CAD build for the part. Positions are in the model's coordinates, mm. Face numbers are marked on the shaded views. A direction names the side the tool comes from. Round coordinates to 2 decimals unless told otherwise and drop trailing zeros. Order: outer loops, then holes, each group sorted by start corner. A loop starts at its lowest first (then second) coordinate and runs counter-clockwise, first axis right, second up. Notation, with made-up numbers: M 8,26.5 L 22,26.5 A20 ccw 22,49.5 Z; hole C -35,39.5 d2. An arc over 180 degrees is marked long. Put each result on its own line as item: value.
```python
from build123d import *

# Parameters (mm, degrees)
SKETCH1_R           = 63.5
BOSS_EXTRUDE1_DEPTH = 14.973360437
SKETCH2_W           = 12.5
SKETCH2_H           = 12.56
CUT_EXTRUDE1_DEPTH  = 10
CIRPATTERN1_COUNT   = 16


with BuildPart() as part:
    # Sketch1 → Boss-Extrude1 (new body)
    with BuildSketch(Plane(origin=(0, 0, 0), x_dir=(1, 0, 0), z_dir=(0, 1, 0))):
        Circle(SKETCH1_R)
    extrude(amount=BOSS_EXTRUDE1_DEPTH)

    # Sketch2 → Cut-Extrude1 (cut)
    with BuildSketch(Plane(origin=(0, 14.973360437, 0), x_dir=(1, 0, 0), z_dir=(0, 1, 0))):
        with Locations((0, -50)):
            Rectangle(SKETCH2_W, SKETCH2_H)
    cut_extrude1 = extrude(amount=-CUT_EXTRUDE1_DEPTH, mode=Mode.SUBTRACT)

    # CirPattern1: Cut-Extrude1 ×16 about axis
    cirpattern1_axis = Axis((0, 0, 0), (0, 1, 0))
    for i in range(1, CIRPATTERN1_COUNT):
        add(cut_extrude1.rotate(cirpattern1_axis, i * 360 / CIRPATTERN1_COUNT), mode=Mode.SUBTRACT)


solid = part.part
```
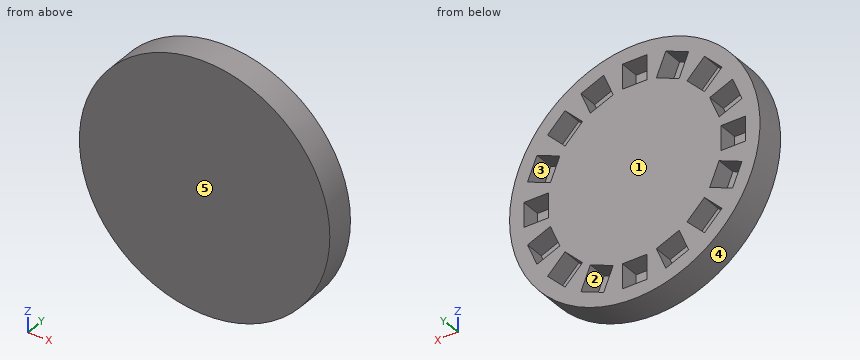
Item 1: Band-saw the part on C-C on y = 11.25. State how many separate pieces and enclosed holes the cut face has, and give its area (3 significant figures).
Answers below:
separate pieces: 1
enclosed holes: 16
area: 10,200 mm²
Item 2: Band-saw the part on A-A on x = 0. Give the cut face in (y, z), and give its area (3 significant figures).
Answers below:
outline: M 0,-63.5 L 14.97,-63.5 L 14.97,-56.28 L 4.97,-56.28 L 4.97,-43.72 L 14.97,-43.72 L 14.97,43.72 L 4.97,43.72 L 4.97,56.28 L 14.97,56.28 L 14.97,63.5 L 0,63.5 Z
area: 1,650 mm²
Item 3: Pin check, flat tips, straight feed: P1, Ø8, axis at x = -42.5, y = 5.5, coming from the -Z side; P2, Ø1, axis at y = 9.5, z = -46, coming from the -X side; P3, Ø5, axis at y = 6.5, z = -47.5, coming from the -X side. Stop position of each tip, or through.
Answers below:
P1: z = -50.5
P2: x = -44.29
P3: x = -44.8
Item 4: Tool access for the marked faces 1 and 2: list every direction of +Z, -Z, +X, -X, +Y, -Y with a clear straight run to the whole face (end or side of a thin tool).
Answers below:
face 1: +Z, -Z, +X, -X, +Y
face 2: +Y
Item 5: Band-saw the part on D-D on y = 3. Give the cut face in (x, z), and give its area (3 significant figures).
Answers below:
outline: C 0,0 d127
area: 12,700 mm²
Item 6: Band-saw the part on B-B on z = 0. Give the cut face in (x, y), and give its area (3 significant figures).
Answers below:
outline: M -63.5,0 L 63.5,0 L 63.5,14.97 L 56.28,14.97 L 56.28,4.97 L 43.72,4.97 L 43.72,14.97 L -43.72,14.97 L -43.72,4.97 L -56.28,4.97 L -56.28,14.97 L -63.5,14.97 Z
area: 1,650 mm²
Item 7: Probe line 1 along Z through (x, y) = (0.5, 9.25); line 2 along Z through (x, y) = (45, 13); line 3 along X through (y, z) = (5.75, 12). List the from-to ranges inside material, lowest first. Write a range as [from, to].
Answers below:
line 1: [-63.5, -56.28], [-43.72, 43.72], [56.28, 63.5]
line 2: [-44.8, -25.4], [-11.87, -6.25], [6.25, 11.87], [25.4, 44.8]
line 3: [-62.36, -45.3], [-42.35, 42.35], [45.3, 62.36]
Item 8: Mould opens along X. For the marked faces 3, 4 and 5 say: pulls with the +X half, pulls with the -X half, needs draft (parallel to the pull), parting line crosses it, or undercut.
Answers below:
face 3: undercut
face 4: parting line crosses it
face 5: needs draft
